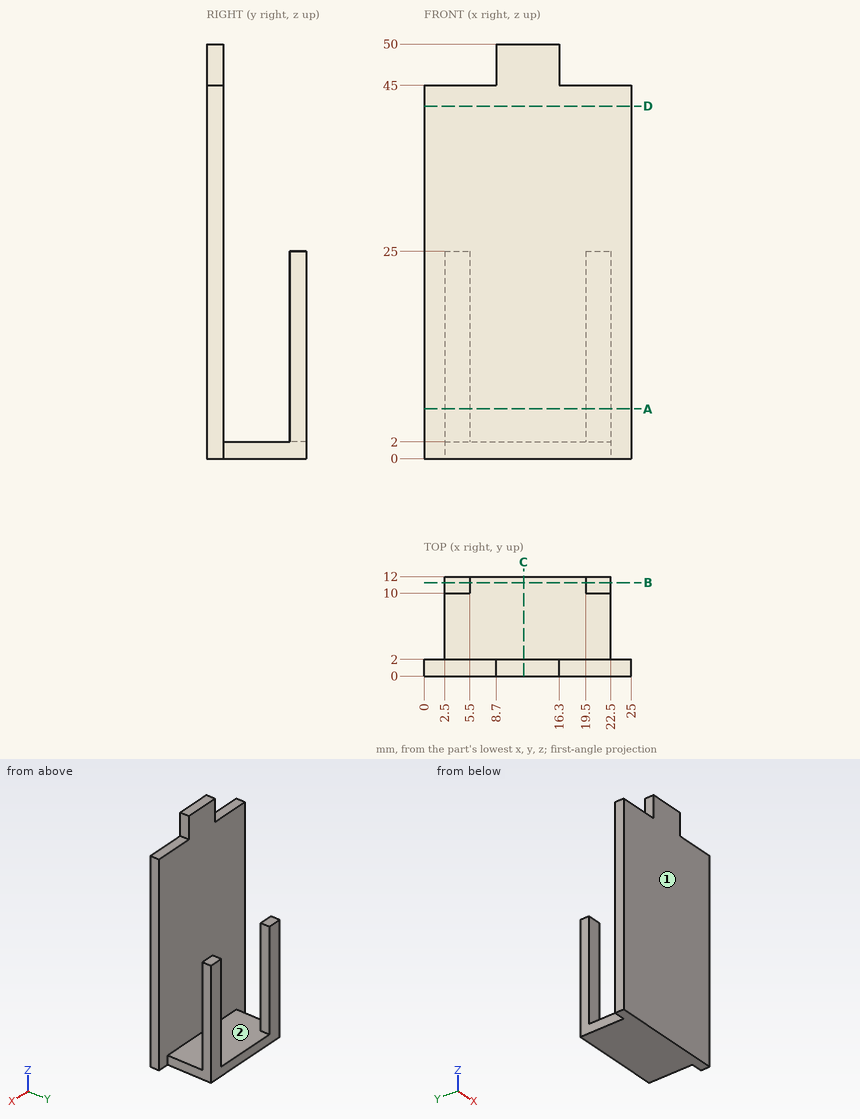
For this review, use the dimensioned drawing (mm, ordinates from the lowest corner) and the shaded views. Round coordinates to 2 decimals unless told otherwise and drop trailing zeros. Order: outer loops, then holes, each group sorted by start corner. A loop starts at its lowest first (then second) coordinate and runs counter-clockwise, first axis right, second up. Notation, with made-up numbers: (-40, 85.25) -> (-2, 85.25) arc R9 cw to (-2, 94.25) -> close; hole circle Ø8 at (23.25, 75.5). An arc over 180 degrees is marked (long way). Use CSV: the item, a comma, the result in double quotes. Start each with the question number.
(1) Mouldability with a two-part tool opening along X and no side actions: class the marked faces 1 and 2 as pulls with the +X half, pulls with the -X half, needs draft (parallel to the pull), parting line crosses it, or undercut.
(2) Consider section B-B on y = 11.25. Write out the cut boundary in (x, z).
(3) Wall thickness on probe 1 along Y at (x, z) = (4, 21); probe 2 along Y at (x, z) = (18.25, 40); probe 3 along Z at (x, y) = (21, 1.5): over which ranges is each line inside the solid? List them lowest first. Write a range as from..to.
(4) Consider section A-A on z = 6. Write out the cut boundary in (x, y), and give its area (3 significant figures).
(5) Consider section D-D on z = 42.5. Write out the cut boundary in (x, y), and give its area (3 significant figures).
(6) Insertion check: pin 1 (4 mm diameter, centred on x = 11, z = 25, fed in from -Y); pin 2 (1.6 mm diameter, centred on y = 10.5, z = 13, fed in from -X); pin 3 (1.6 mm diameter, centred on x = 6, y = 0.5, fed in from +Z); pin 4 (1.5 mm diameter, centred on x = 19.5, z = 32.5, fed in from +Y). Each pin has a flat end and moves straight along its axis. Give the tip position at first contact, or say it passes through.
(7) Consider section C-C on x = 12. Write out the cut boundary in (y, z).
Responses:
1,face 1,"needs draft"
1,face 2,"undercut"
2,outline,"(2.5, 0) -> (22.5, 0) -> (22.5, 25) -> (19.5, 25) -> (19.5, 2) -> (5.5, 2) -> (5.5, 25) -> (2.5, 25) -> close"
3,probe 1,"0..2, 10..12"
3,probe 2,"0..2"
3,probe 3,"0..45"
4,outline,"(0, 0) -> (25, 0) -> (25, 2) -> (0, 2) -> close; (2.5, 10) -> (5.5, 10) -> (5.5, 12) -> (2.5, 12) -> close; (19.5, 10) -> (22.5, 10) -> (22.5, 12) -> (19.5, 12) -> close"
4,area,"62.0 mm²"
5,outline,"(0, 0) -> (25, 0) -> (25, 2) -> (0, 2) -> close"
5,area,"50.0 mm²"
6,pin 1,"y = 0"
6,pin 2,"x = 2.5"
6,pin 3,"z = 45"
6,pin 4,"y = 2"
7,outline,"(0, 0) -> (12, 0) -> (12, 2) -> (2, 2) -> (2, 50) -> (0, 50) -> close"
